Verification items for the finished model (mm, model axes). Give positions to 0.01 mm unless a question says otherwise; leave off trailing zeros. Write each loop counter-clockwise with the first axis right and the second up, starting at its lowest first coordinate (ties: lowest second). Pieces come first, ordered by that corner, then holes. Notation, with made-up numbers: (-28.75, 26) - (8.25, 26) arc R12 ccw to (8.25, 36) - close; hole circle Ø6 at (77.5, 29). An arc over 180 degrees is marked (long way). Answer as a JSON object with one key per item and string values. Group by question number.
Item 1: Scan lines: line 1 along X through (y, z) = (0.75, -61.75); line 2 along Z through (x, y) = (74.5, 0.7); line 3 along X through (y, z) = (1.95, -32). Record each from-to range of solid material in increasing order. Write a range as [from, to].
Item 2: Sectioned sample at C-C, the plane y = 0.7. Count the separate pieces of the cut face and the enclosed holes in it, and give its area (3 significant figures).
Item 3: Sectioned sample at D-D, the plane z = -55.5. Record the boundary of the cut face in (x, y).
Item 4: Go/stop test with a flat-tipped pin: pin 1 (5 mm diameter, centred on x = 28, z = -61.75, fed in from +Y). Record where the tip stops, or that it passes through.
Item 5: Sectioned sample at A-A, the plane x = 76. Record the boundary of the cut face in (y, z), and give its area (3 significant figures).
Item 6: Sectioned sample at B-B, the plane z = -46.5. Record the boundary of the cut face in (x, y), and give its area (3 significant figures).
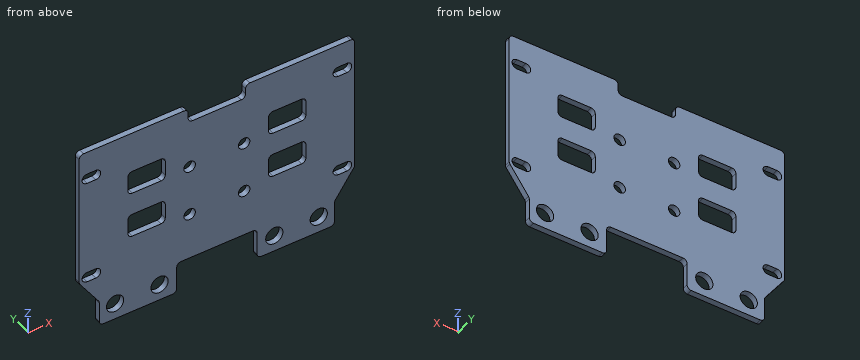
```python
from build123d import *

# Parameters (mm, degrees)
SKETCH1_R           = 2
SKETCH1_R_2         = 3
SKETCH1_W           = 13
SKETCH1_H           = 8.25
BOSS_EXTRUDE1_DEPTH = 2
FILLET1_R           = 1.5


with BuildPart() as part:
    # Sketch1 → Boss-Extrude1 (new body)
    with BuildSketch(Plane(origin=(0, 0, 0), x_dir=(1, 0, 0), z_dir=(0, 1, 0))):
        Polygon((38, 0), (38, 5), (58, 5), (58, 0), (96, 0), (96, 48.5), (89, 58.5), (89, 67.5), (62, 67.5), (62, 56.5), (34, 56.5), (34, 67.5), (7, 67.5), (7, 58.5), (0, 48.5), (0, 0), align=None)
        with Locations(Location((38.5, 40, 0), (0, 0, 270))):
            Circle(SKETCH1_R, mode=Mode.SUBTRACT)
        with Locations(Location((38.5, 22, 0), (0, 0, 270))):
            Circle(SKETCH1_R, mode=Mode.SUBTRACT)
        with Locations(Location((57.5, 22, 0), (0, 0, 90))):
            Circle(SKETCH1_R, mode=Mode.SUBTRACT)
        with Locations(Location((57.5, 40, 0), (0, 0, 90))):
            Circle(SKETCH1_R, mode=Mode.SUBTRACT)
        with Locations(Location((12.5, 61.75, 0), (0, 0, 270))):
            Circle(SKETCH1_R_2, mode=Mode.SUBTRACT)
        with Locations(Location((28, 61.75, 0), (0, 0, 270))):
            Circle(SKETCH1_R_2, mode=Mode.SUBTRACT)
        with Locations(Location((68, 61.75, 0), (0, 0, 90))):
            Circle(SKETCH1_R_2, mode=Mode.SUBTRACT)
        with Locations(Location((83.5, 61.75, 0), (0, 0, 90))):
            Circle(SKETCH1_R_2, mode=Mode.SUBTRACT)
        with Locations((72.5, 18.625)):
            Rectangle(SKETCH1_W, SKETCH1_H, mode=Mode.SUBTRACT)
        with Locations((23.5, 34.875)):
            Rectangle(SKETCH1_W, SKETCH1_H, mode=Mode.SUBTRACT)
        with Locations((23.5, 18.625)):
            Rectangle(SKETCH1_W, SKETCH1_H, mode=Mode.SUBTRACT)
        with Locations((72.5, 34.875)):
            Rectangle(SKETCH1_W, SKETCH1_H, mode=Mode.SUBTRACT)
        with BuildLine():
            Line((2.75, 11.75), (5.75, 11.75))
            ThreePointArc((5.75, 11.75), (7.5, 10), (5.75, 8.25))
            Line((5.75, 8.25), (2.75, 8.25))
            ThreePointArc((2.75, 8.25), (1, 10), (2.75, 11.75))
        make_face(mode=Mode.SUBTRACT)
        with BuildLine():
            Line((93.25, 8.25), (90.25, 8.25))
            ThreePointArc((90.25, 8.25), (88.5, 10), (90.25, 11.75))
            Line((90.25, 11.75), (93.25, 11.75))
            ThreePointArc((93.25, 11.75), (95, 10), (93.25, 8.25))
        make_face(mode=Mode.SUBTRACT)
        with BuildLine():
            Line((93.25, 45.5), (90.25, 45.5))
            ThreePointArc((90.25, 45.5), (88.5, 47.25), (90.25, 49))
            Line((90.25, 49), (93.25, 49))
            ThreePointArc((93.25, 49), (95, 47.25), (93.25, 45.5))
        make_face(mode=Mode.SUBTRACT)
        with BuildLine():
            Line((2.75, 49), (5.75, 49))
            ThreePointArc((5.75, 49), (7.5, 47.25), (5.75, 45.5))
            Line((5.75, 45.5), (2.75, 45.5))
            ThreePointArc((2.75, 45.5), (1, 47.25), (2.75, 49))
        make_face(mode=Mode.SUBTRACT)
    extrude(amount=BOSS_EXTRUDE1_DEPTH)

    # Fillet1
    fillet1_edges = [part.edges().sort_by_distance(p)[0] for p in [
        (0, 1, -48.5),
        (7, 1, -58.5),
        (7, 1, -67.5),
        (34, 1, -67.5),
        (34, 1, -56.5),
        (62, 1, -56.5),
        (62, 1, -67.5),
        (89, 1, -67.5),
        (89, 1, -58.5),
        (96, 1, -48.5),
        (96, 1, 0),
        (58, 1, 0),
        (58, 1, -5),
        (38, 1, -5),
        (38, 1, 0),
        (0, 1, 0),
        (17, 1, -39),
        (17, 1, -30.75),
        (30, 1, -30.75),
        (30, 1, -39),
        (17, 1, -22.75),
        (17, 1, -14.5),
        (30, 1, -14.5),
        (30, 1, -22.75),
        (79, 1, -14.5),
        (79, 1, -22.75),
        (66, 1, -22.75),
        (66, 1, -14.5),
        (79, 1, -30.75),
        (79, 1, -39),
        (66, 1, -39),
        (66, 1, -30.75),
    ]]
    fillet(fillet1_edges, radius=FILLET1_R)


solid = part.part
```
Geometry check:
{
 "1": {"line 1": "[7, 9.5], [15.5, 25], [31, 34], [62, 65], [71, 80.5], [86.5, 89]", "line 2": "[-67.5, -39], [-30.75, -22.75], [-14.5, 0]", "line 3": "[0, 17.02], [29.98, 66.02], [78.98, 96]"},
 "2": {"separate pieces": "1", "enclosed holes": "16", "area": "5,210 mm^2"},
 "3": {"outline": "(4.9, 0) - (91.1, 0) - (91.1, 2) - (4.9, 2) - close"},
 "4": {"pin 1": "through"},
 "5": {"outline": "(0, -67.5) - (2, -67.5) - (2, -39) - (0, -39) - close; (0, -30.75) - (2, -30.75) - (2, -22.75) - (0, -22.75) - close; (0, -14.5) - (2, -14.5) - (2, 0) - (0, 0) - close", "area": "102 mm^2"},
 "6": {"outline": "(0, 0) - (1.17, 0) - (1.17, 2) - (0, 2) - close; (7.33, 0) - (88.67, 0) - (88.67, 2) - (7.33, 2) - close; (94.83, 0) - (96, 0) - (96, 2) - (94.83, 2) - close", "area": "167 mm^2"}
}
